Input: part model. Units: mm. Frame: model coordinates. Face numbers are marked on the shaded views. A direction names the side the tool comes from. Round coordinates to 2 decimals unless told otherwise and drop trailing zeros. Loops run counter-clockwise (first coordinate to the right, second up) from the corner with the lowest first, then second, coordinate; pieces in that order, holes last. Notation, with made-up numbers: (60.25, 89) -> (81.25, 89) arc R21 ccw to (81.25, 102) -> close; hole circle Ø5 at (22, 21.5). An arc over 180 degrees is marked (long way). Answer as a JSON object with one key per item and string values.
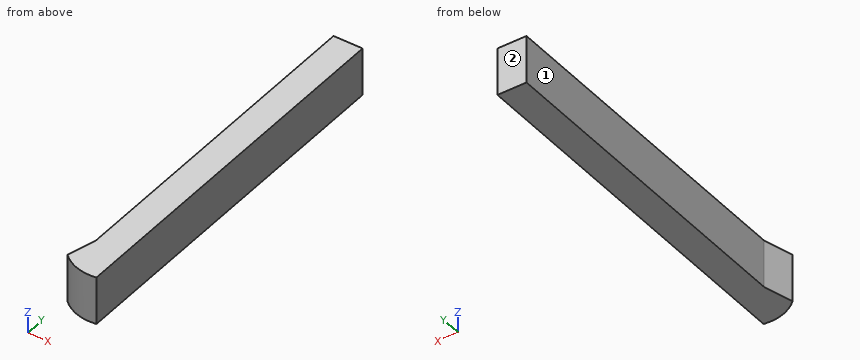
```python
from build123d import *

# Parameters (mm, degrees)
F0_W     = 15.477344
F0_H     = 72.370944
F1_DEPTH = 25.4


with BuildPart() as f1:
    # F0 (on Top) → F1 (new body)
    with BuildSketch(Plane.XY):
        with BuildLine():
            Line((-15.477344, -142.19746), (-15.477344, -130.952388))
            Line((-15.477344, -130.952388), (-19.745878, -146.344457))
            ThreePointArc((-19.745878, -146.344457), (-10.60441, -151.765249), (0, -152.470872))
            Line((0, -152.470872), (0, -142.19746))
            Line((0, -142.19746), (-15.477344, -142.19746))
        make_face()
        Polygon((0, -23.784393), (-15.477344, -23.784393), (-15.477344, -130.952388), (-15.477344, -142.19746), (0, -142.19746), align=None)
        with Locations((-7.738672, 12.401079)):
            Rectangle(F0_W, F0_H)
    extrude(amount=F1_DEPTH)


solid = f1.part
```
1) Reachability of the marked faces 1 and 2 from +Z, -Z, +X, -X, +Y, -Y: full face, straight path, thin tool, end or side. Return the list, or none.
Output:
{"face 1": "+Z, -Z, -X, +Y", "face 2": "+Z, -Z, +X, -X, +Y"}
2) Section A-A, the plane z = 2.75. Output: boundary loops of the cut face in (x, y).
Output:
{"outline": "(-19.75, -146.34) arc R22.88 ccw to (0, -152.47) -> (0, 48.59) -> (-15.48, 48.59) -> (-15.48, -130.95) -> close"}
3) Ray query, probe 1 along Y at (x, z) = (-4.5, 17); probe 2 along X at (y, z) = (-130.5, 5.75); probe 3 along Y at (x, z) = (-2, 10.75). Return the intervals inside material, ascending.
Output:
{"probe 1": "y = -152.78 to 48.59", "probe 2": "x = -15.48 to 0", "probe 3": "y = -152.72 to 48.59"}
4) Section B-B, the plane y = -86. Output: boundary loops of the cut face in (x, z).
Output:
{"outline": "(-15.48, 0) -> (0, 0) -> (0, 25.4) -> (-15.48, 25.4) -> close"}
5) Contact query for flat-ended pins moving along their axis: P1, Ø12.5, axis at y = -47, z = 11, coming from the -X side; P2, Ø2, axis at x = -5.5, z = 19.5, coming from the -Y side; P3, Ø8, axis at x = -11, z = 12, coming from the -Y side. Output: stop coordinate, or through.
Output:
{"P1": "stops at x = -15.48", "P2": "stops at y = -152.78", "P3": "stops at y = -152.57"}
